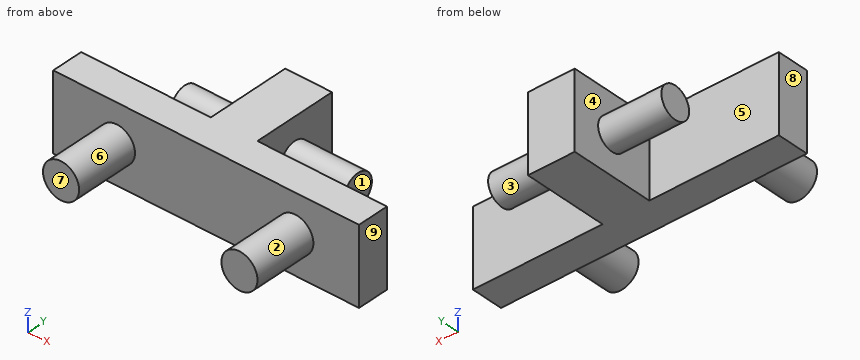
from build123d import *

# Parameters (mm, degrees)
F0_W     = 27.94
F0_H     = 45.72
F1_DEPTH = 19.05
F2_W     = 27.94
F2_H     = 45.72
F3_DEPTH = 50.8
F5_R     = 9.4615
F6_DEPTH = 37.846
F7_DEPTH = 37.846
F9_DEPTH = 38.1


with BuildPart() as f1:
    # F0 (on Front) → F1 (new body)
    with BuildSketch(Plane.XZ):
        Polygon((-8.658381, 40.910337), (-74.698381, 40.910337), (-74.698381, -4.809663), (2.771619, -4.809663), (2.771619, 40.910337), align=None)
        with Locations((16.741619, 18.050337)):
            Rectangle(F0_W, F0_H)
        Polygon((42.141619, 40.910337), (30.711619, 40.910337), (30.711619, -4.809663), (108.181619, -4.809663), (108.181619, 40.910337), align=None)
    extrude(amount=F1_DEPTH)

    # F2 (on face) → F3 (join)
    with BuildSketch(Plane(origin=(0, 0, 0), x_dir=(-1, 0, 0), z_dir=(0, 1, 0))):
        with Locations((-16.741619, 18.050337)):
            Rectangle(F2_W, F2_H)
    extrude(amount=F3_DEPTH)

    # F5 (on face) → F6 (join)
    with BuildSketch(Plane.YZ.offset(30.711619)):
        with Locations((25.4, 18.050337)):
            Circle(F5_R)
    extrude(amount=F6_DEPTH)

    # F4 (on face) → F7 (join)
    with BuildSketch(Plane(origin=(2.771619, 0, 0), x_dir=(0, -1, 0), z_dir=(-1, 0, 0))):
        with BuildLine():
            ThreePointArc((-34.8615, 18.050337), (-25.4, 8.588837), (-15.9385, 18.050337))
            ThreePointArc((-15.9385, 18.050337), (-25.4, 27.511837), (-34.8615, 18.050337))
        make_face()
    extrude(amount=F7_DEPTH)

    # F8 (on face) → F9 (join)
    with BuildSketch(Plane.XZ.offset(19.05)):
        with BuildLine():
            Line((-47.393381, 18.050337), (-36.598381, 18.050337))
            Line((-36.598381, 18.050337), (-25.803381, 18.050337))
            ThreePointArc((-25.803381, 18.050337), (-36.598381, 28.845337), (-47.393381, 18.050337))
        make_face()
        with BuildLine():
            Line((-25.803381, 18.050337), (-36.598381, 18.050337))
            Line((-36.598381, 18.050337), (-47.393381, 18.050337))
            ThreePointArc((-47.393381, 18.050337), (-36.598381, 7.255337), (-25.803381, 18.050337))
        make_face()
        with BuildLine():
            ThreePointArc((80.876619, 18.050337), (70.081619, 28.845337), (59.286619, 18.050337))
            Line((59.286619, 18.050337), (70.081619, 18.050337))
            Line((70.081619, 18.050337), (80.876619, 18.050337))
        make_face()
        with BuildLine():
            Line((70.081619, 18.050337), (59.286619, 18.050337))
            ThreePointArc((59.286619, 18.050337), (70.081619, 7.255337), (80.876619, 18.050337))
            Line((80.876619, 18.050337), (70.081619, 18.050337))
        make_face()
    extrude(amount=F9_DEPTH)


solid = f1.part
Verification items for the finished model (mm, model axes). Face numbers are marked on the shaded views. A direction names the side the tool comes from. Give positions to 0.01 mm unless a question says otherwise; leave off trailing zeros. Write each loop counter-clockwise with the first axis right and the second up, starting at its lowest first coordinate (ties: lowest second). Pieces come first, ordered by that corner, then holes. Notation, with made-up numbers: M 14,-2 L 37,-2 A21 ccw 37,9 Z; hole C -36.75,85 d1. An arc over 180 degrees is marked long. Use CSV: the item, a comma, the result in double quotes.
1) Material ranges on line 1 along X through (y, z) = (39, -2.5); line 2 along Y through (x, z) = (27.5, 27); line 3 along Y through (x, z) = (97, 33), recorded low to high.
Final values:
line 1,"2.77 to 30.71"
line 2,"-19.05 to 50.8"
line 3,"-19.05 to 0"
2) Cross-section at A-A (x = 64). Enter the section's corners in (y, z), plus the area to 3 significant figures.
Final values:
outline,"M -57.15,9.13 L -19.05,9.13 L -19.05,-4.81 L 0,-4.81 L 0,40.91 L -19.05,40.91 L -19.05,26.97 L -57.15,26.97 Z; C 25.4,18.05 d18.92"
area,"1,830 mm²"
3) Cross-section at C-C (y = 25.4). Enter the section's corners in (x, z), plus the area to 3 significant figures.
Final values:
outline,"M -35.07,8.59 L 2.77,8.59 L 2.77,-4.81 L 30.71,-4.81 L 30.71,8.59 L 68.56,8.59 L 68.56,27.51 L 30.71,27.51 L 30.71,40.91 L 2.77,40.91 L 2.77,27.51 L -35.07,27.51 Z"
area,"2,710 mm²"
4) Go/stop test with flat-tipped pins: pin 1 Ø9.5 at (y, z) = (22.5, 19.5) entering from -X; pin 2 Ø6 at (x, z) = (-41, 0.5) entering from -Y; pin 3 Ø4 at (y, z) = (37.5, 16) entering from -X. Record where each tip stops, or that it passes through.
Final values:
pin 1,"x = -35.07"
pin 2,"y = -19.05"
pin 3,"x = 2.77"
5) Release check for a two-part mould opening along X. For the marked faces 6, 7, 8 and 9 record: released by +X, released by -X, zero draft, split by the parting line, or undercut.
Final values:
face 6,"undercut"
face 7,"zero draft"
face 8,"released by -X"
face 9,"released by +X"
6) Cross-section at B-B (z = 4). Enter the section's corners in (x, y).
Final values:
outline,"M -74.7,-19.05 L 108.18,-19.05 L 108.18,0 L 30.71,0 L 30.71,50.8 L 2.77,50.8 L 2.77,0 L -74.7,0 Z"
7) Access from +Z, -Z, +X, -X, +Y, -Y to the whole of each face (thin tool, end or side, straight path). Record for the marked faces 1, 2, 3, 4 and 5.
Final values:
face 1,"+Z, -Z, +X, +Y"
face 2,"-Y"
face 3,"+X"
face 4,"-X"
face 5,"+Z, -Z, -X"
8) Cross-section at D-D (y = -42.5). Enter the section's corners in (x, z) (3 decimals).
Final values:
outline,"C -36.598,18.05 d21.59; C 70.082,18.05 d21.59"
